Check sheet for the modelled part. Datum: model origin and axes. Units: mm. Face numbers are marked on the shaded views. A direction names the side the tool comes from. Give positions to 0.01 mm unless a question says otherwise; leave off trailing zeros. Order: outer loops, then holes, each group sorted by start corner. A loop starts at its lowest first (then second) coordinate and runs counter-clockwise, first axis right, second up. Notation, with made-up numbers: (-37.75, 38) - (-3.75, 38) arc R16 ccw to (-3.75, 46) - close; hole circle Ø5 at (34, -19.5). An arc over 180 degrees is marked (long way). Answer in a Markdown table with one row per item.
from build123d import *

# Parameters (mm, degrees)
F1_DEPTH  = 15
F2_R      = 3
F2_R_2    = 9
F3_DEPTH  = 15.001
F4_R      = 5.5
F5_DEPTH  = 6
F6_R      = 10.25
F7_DEPTH  = 12
F9_D      = 5
F9_DEPTH  = 35
F10_R     = 5
F10_R_2   = 2.5
F11_DEPTH = 18
F12_R     = 3
F12_R_2   = 2.5
F13_DEPTH = 17.9


with BuildPart() as f1:
    # F0 (on Top) → F1 (new body)
    with BuildSketch(Plane.XY):
        Polygon((0, 127), (0, 0), (75, 0), (75, 98), (55, 98), (55, 127), align=None)
    extrude(amount=F1_DEPTH)

    # F2 (on face) → F3 (cut, through all)
    with BuildSketch(Plane(origin=(0, 0, 0), x_dir=(1, 0, 0), z_dir=(0, 0, -1))):
        with Locations((5, -121)):
            Circle(F2_R)
        with Locations((5, -83)):
            Circle(F2_R)
        with Locations((41, -60)):
            Circle(F2_R_2)
        with Locations((67.5, -24)):
            Circle(F2_R)
        with Locations((67.5, -74)):
            Circle(F2_R)
    extrude(amount=-F3_DEPTH, mode=Mode.SUBTRACT)

    # F4 (on face) → F5 (cut)
    with BuildSketch(Plane(origin=(0, 0, 0), x_dir=(1, 0, 0), z_dir=(0, 0, -1))):
        with Locations((67.5, -74)):
            Circle(F4_R)
        with Locations((67.5, -24)):
            Circle(F4_R)
    extrude(amount=-F5_DEPTH, mode=Mode.SUBTRACT)

    # F6 (on face) → F7 (cut)
    with BuildSketch(Plane.XY.offset(15)):
        with Locations((41, 100)):
            Circle(F6_R)
        with Locations((41, 20)):
            Circle(F6_R)
    extrude(amount=-F7_DEPTH, mode=Mode.SUBTRACT)

    # F9
    with Locations(Plane(origin=(0, 0, 0), x_dir=(0, -1, 0), z_dir=(-1, 0, 0))):
        with Locations((-100, 7.5), (-20, 7.5)):
            Hole(F9_D / 2, depth=F9_DEPTH)

    # F10 (on face) → F11 (cut)
    with BuildSketch(Plane(origin=(0, 0, 0), x_dir=(0, -1, 0), z_dir=(-1, 0, 0))):
        with Locations((-100, 7.5)):
            Circle(F10_R)
        with Locations((-100, 7.5)):
            Circle(F10_R_2, mode=Mode.SUBTRACT)
        with Locations((-20, 7.5)):
            Circle(F10_R)
        with Locations((-20, 7.5)):
            Circle(F10_R_2, mode=Mode.SUBTRACT)
    extrude(amount=-F11_DEPTH, mode=Mode.SUBTRACT)

    # F12 (on face) → F13 (cut)
    with BuildSketch(Plane.XZ):
        with Locations((64, 7.5)):
            Circle(F12_R)
        with Locations((10, 7.5)):
            Circle(F12_R_2)
    extrude(amount=-F13_DEPTH, mode=Mode.SUBTRACT)


with BuildPart() as f14_1:
    # F14: instance of F1
    add(f1.part.mirror(Plane(origin=(0, 63.814533, 7.5), x_dir=(0, -1, 0), z_dir=(-1, 0, 0))))


solid = f14_1.part
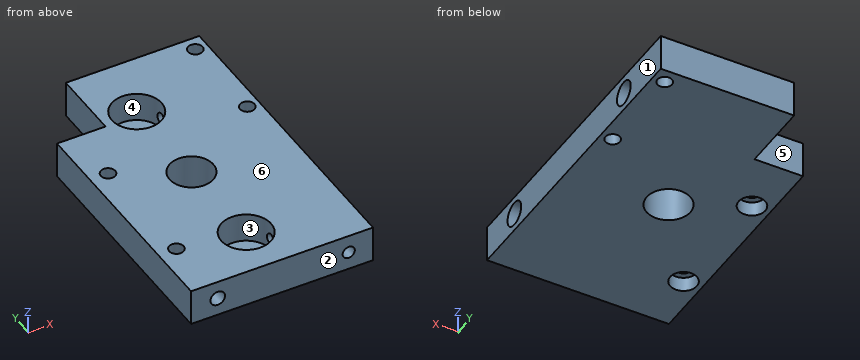
(1) Cross-section at B-B, the plane x = -41. Record the cut outline in (y, z), then the cut area to 3 significant figures.
Geometry says:
| item | result |
|---|---|
| outline | (0, 0) - (51, 0) - (51, 15) - (30.25, 15) - (30.25, 3) - (9.75, 3) - (9.75, 15) - (0, 15) - close; (69, 0) - (127, 0) - (127, 15) - (110.25, 15) - (110.25, 3) - (89.75, 3) - (89.75, 15) - (69, 15) - close |
| area | 1,140 mm² |
(2) Mould release check, pull along X, two halves, no side actions. Record for the marked faces 1, 2 and 3: pulls with the +X half, pulls with the -X half, needs draft (parallel to the pull), parting line crosses it, or undercut.
Geometry says:
| item | result |
|---|---|
| face 1 | pulls with the +X half |
| face 2 | needs draft |
| face 3 | undercut |
(3) Access from +Z, -Z, +X, -X, +Y, -Y to the whole of each face (thin tool, end or side, straight path). Record for the marked faces 4, 5 and 6.
Geometry says:
| item | result |
|---|---|
| face 4 | +Z |
| face 5 | +Z, -Z, -X, +Y |
| face 6 | +Z, +X, -X, +Y, -Y |
(4) Gauge pin test, flat ends, axial feed: P1, Ø5.5, axis at x = -64, z = 7.5, coming from the -Y side; P2, Ø6.5, axis at x = -67.5, y = 74, coming from the -Z side; P3, Ø5, axis at y = 98, z = 7, coming from the +X side. Record the tip position at first contact, or that the pin passes through.
Geometry says:
| item | result |
|---|---|
| P1 | y = 17.9 |
| P2 | z = 6 |
| P3 | x = -18 |
(5) Cross-section at D-D, the plane z = 7.5. Give the number of separate pieces and of enclosed holes in the cut face, then the cut area to 3 significant figures.
Geometry says:
| item | result |
|---|---|
| separate pieces | 2 |
| enclosed holes | 5 |
| area | 7,250 mm² |
(6) Cross-section at C-C, the plane x = -21. Record the cut outline in (y, z), then the cut area to 3 significant figures.
Geometry says:
| item | result |
|---|---|
| outline | (0, 0) - (127, 0) - (127, 15) - (0, 15) - close; hole circle Ø5 at (20, 7.5); hole circle Ø5 at (100, 7.5) |
| area | 1,870 mm² |
(7) Cross-section at A-A, the plane y = 74. Record the cut outline in (x, z), then the cut area to 4 significant figures.
Geometry says:
| item | result |
|---|---|
| outline | (-75, 0) - (-73, 0) - (-73, 6) - (-70.5, 6) - (-70.5, 15) - (-75, 15) - close; (-64.5, 6) - (-62, 6) - (-62, 0) - (0, 0) - (0, 15) - (-64.5, 15) - close |
| area | 1,005 mm² |
(8) Thickness scan on L1, parallel to Y at x = -41, z = 12.5; L2, parallel to Y at x = -67.5, z = 9; L3, parallel to Y at x = -67.5, z = 2.45. Record the ranges inside material, lowest first.
Geometry says:
| item | result |
|---|---|
| L1 | 0 to 9.75, 30.25 to 51, 69 to 89.75, 110.25 to 127 |
| L2 | 0 to 21, 27 to 71, 77 to 98 |
| L3 | 0 to 18.5, 29.5 to 68.5, 79.5 to 98 |
